from build123d import *

# Parameters (mm, degrees)
F1_DEPTH = 11
F2_DEPTH = 8
F3_DEPTH = 4.5


# Not quite as in the source:
# - ends of sketch curves that miss each other by under 0.0002 mm in the source are joined
# - a feature names something its author has since deleted; it is built from what else it names


with BuildPart() as f1:
    # F0 (on Top) → F1 (new body)
    with BuildSketch(Plane.XY):
        with BuildLine():
            ThreePointArc((-3.905e-06, -110), (9.5871245695, -109.5814174141), (19.1012892866, -108.3288546399))
            Line((19.1012892866, -108.3288546399), (18.1462248222, -102.9124119079))
            ThreePointArc((18.1462248222, -102.9124119079), (9.107768341, -104.1023465434), (-3.7098e-06, -104.5))
            Line((-3.7098e-06, -104.5), (-3.905e-06, -110))
        make_face()
        with BuildLine():
            Line((-18.1462345662, -102.9124101898), (-19.1012995434, -108.3288528313))
            ThreePointArc((-19.1012995434, -108.3288528313), (-9.5871336473, -109.5814166199), (-3.905e-06, -110))
            Line((-3.905e-06, -110), (-3.7098e-06, -104.5))
            ThreePointArc((-3.7098e-06, -104.5), (-9.107776965, -104.1023457889), (-18.1462345662, -102.9124101898))
        make_face()
    extrude(amount=F1_DEPTH)

    # F0 (on Top) → F2 (join)
    with BuildSketch(Plane.XY):
        with BuildLine():
            Line((-14.1061584567, -80), (-18.1462345662, -102.9124101898))
            ThreePointArc((-18.1462345662, -102.9124101898), (-9.107776965, -104.1023457889), (-3.7098e-06, -104.5))
            Line((-3.7098e-06, -104.5), (-3.673e-06, -103.4654280496))
            ThreePointArc((-3.673e-06, -103.4654280496), (-3.8705432222, -101.8678665034), (-5.4745569582, -97.999996388))
            Line((-5.4745569582, -97.999996388), (-5.4745569582, -85.9715496865))
            ThreePointArc((-5.4745569582, -85.9715496865), (-3.6975375335, -82.4283616447), (-2.8755e-06, -81))
            Line((-2.8755e-06, -81), (-2.84e-06, -80))
            Line((-2.84e-06, -80), (-14.1061584567, -80))
        make_face()
        with BuildLine():
            ThreePointArc((-3.7098e-06, -104.5), (9.107768341, -104.1023465434), (18.1462248222, -102.9124119079))
            Line((18.1462248222, -102.9124119079), (14.1061506466, -80))
            Line((14.1061506466, -80), (-2.84e-06, -80))
            Line((-2.84e-06, -80), (-2.8755e-06, -81))
            ThreePointArc((-2.8755e-06, -81), (3.6975315365, -82.4283617759), (5.4745508166, -85.9715496865))
            Line((5.4745508166, -85.9715496865), (5.4563215634, -97.999996388))
            ThreePointArc((5.4563215634, -97.999996388), (3.8587524181, -101.8614219128), (-3.673e-06, -103.4654280496))
            Line((-3.673e-06, -103.4654280496), (-3.7098e-06, -104.5))
        make_face()
    extrude(amount=F2_DEPTH)

    # F0 (on Top) → F3 (join)
    with BuildSketch(Plane.XY):
        with BuildLine():
            ThreePointArc((-5.4745569582, -97.999996388), (-3.8705432222, -101.8678665034), (-3.673e-06, -103.4654280496))
            Line((-3.673e-06, -103.4654280496), (-3.5722e-06, -100.6249805656))
            ThreePointArc((-3.5722e-06, -100.6249805656), (-1.862784569, -99.858636786), (-2.6341168729, -97.9979158754))
            Line((-2.6341168729, -97.9979158754), (-2.6250022463, -86.4979194874))
            ThreePointArc((-2.6250022463, -86.4979194874), (-1.8554226203, -84.6431092399), (-2.9776e-06, -83.875))
            Line((-2.9776e-06, -83.875), (-2.8755e-06, -81))
            ThreePointArc((-2.8755e-06, -81), (-3.6975375335, -82.4283616447), (-5.4745569582, -85.9715496865))
            Line((-5.4745569582, -85.9715496865), (-5.4745569582, -97.999996388))
        make_face()
        with BuildLine():
            Line((-3.5722e-06, -100.6249805656), (-3.673e-06, -103.4654280496))
            ThreePointArc((-3.673e-06, -103.4654280496), (3.8587524181, -101.8614219128), (5.4563215634, -97.999996388))
            Line((5.4563215634, -97.999996388), (5.4745508166, -85.9715496865))
            ThreePointArc((5.4745508166, -85.9715496865), (3.6975315365, -82.4283617759), (-2.8755e-06, -81))
            Line((-2.8755e-06, -81), (-2.9776e-06, -83.875))
            ThreePointArc((-2.9776e-06, -83.875), (1.8561522628, -84.6438447323), (2.6249969292, -86.5))
            ThreePointArc((2.6249969292, -86.5), (2.6249967231, -86.5010402564), (2.6249961047, -86.5020805126))
            Line((2.6249961047, -86.5020805126), (2.6158831271, -97.9999963886))
            ThreePointArc((2.6158831271, -97.9999963886), (2.6158820965, -98.0010366444), (2.6158814781, -98.0020769006))
            ThreePointArc((2.6158814781, -98.0020769006), (1.8495227006, -99.8536632596), (-3.5722e-06, -100.6249805656))
        make_face()
    extrude(amount=F3_DEPTH)


solid = f1.part
Geometry: final body of the model. Coordinates: model frame, mm. A direction names the side the tool comes from. Give positions to 0.01 mm unless a question says otherwise; leave off trailing zeros. Write each loop counter-clockwise with the first axis right and the second up, starting at its lowest first coordinate (ties: lowest second). Pieces come first, ordered by that corner, then holes. Notation, with made-up numbers: (28.25, -28.5) - (36.25, -28.5) arc R23 cw to (36.25, -15.5) - close; hole circle Ø5 at (47, -8). An arc over 180 degrees is marked (long way). Return JSON: item names as keys, results as strings. Group by question number.
1) Section A-A on y = -85.5. Return the cut outline in (x, z), plus the area to 3 significant figures.
2) Line query: line 1 (Z direction, x = 12, y = -103.5); line 2 (X direction, y = -100, z = 3.25); line 3 (Z direction, x = 3, y = -94). Output: solid intervals per line, ascending.
3) Set-up query: faces 1 (the flat face through (0, -80, 4)), 2 (the flat face through (8, -92, 8)), 3 (the flat face through (4, -92, 4.5)). Return all of +Z, -Z, +X, -X, +Y, -Y with unobstructed straight access to the full face (end or side cutting, diameter ignored); none if empty.
4) Section C-C on z = 8.5. Return the cut outline in (x, y), plus the area to 3 significant figures.
5) Section D-D on y = -104. Return the cut outline in (x, z), plus the area to 3 significant figures.
6) Section B-B on z = 6.25. Return the cut outline in (x, y), plus the area to 3 significant figures.
7) Mould query, pull axis X, two halves, no side actions, for faces 4 (the flat face through (0, -106, 11)), 5 (the flat face through (-5.475, -92, 6)). Classes: released by +X, released by -X, zero draft, split by the parting line, or undercut.
8) First-contact query: P1, Ø12, axis at x = 1.5, y = -89.5, coming from the +Z side; P2, Ø1, axis at y = -93, z = 8, coming from the +X side; P3, Ø4, axis at y = -92.5, z = 5.5, coming from the +X side; P4, Ø3, axis at y = -92.5, z = 10, coming from the +X side. Flat tips, straight axial feed; report the tip coordinate or a pass-through.
Filled in:
{
 "1": {"outline": "(-15.08, 0) - (-2.43, 0) - (-2.43, 4.5) - (-5.41, 4.5) - (-5.41, 8) - (-15.08, 8) - close; (2.43, 0) - (15.08, 0) - (15.08, 8) - (5.41, 8) - (5.41, 4.5) - (2.43, 4.5) - close", "area": "182 mm^2"},
 "2": {"line 1": "z = 0 to 8", "line 2": "x = -17.63 to -1.71, 1.69 to 17.63", "line 3": "z = 0 to 4.5"},
 "3": {"face 1": "+Z, -Z, +X, -X, +Y", "face 2": "+Z, +Y", "face 3": "+Z"},
 "4": {"outline": "(-19.1, -108.33) arc R110 ccw to (19.1, -108.33) - (18.15, -102.91) arc R104.5 cw to (-18.15, -102.91) - close", "area": "206 mm^2"},
 "5": {"outline": "(-18.34, 0) - (18.34, 0) - (18.34, 11) - (10.21, 11) - (10.21, 8) - (-10.21, 8) - (-10.21, 11) - (-18.34, 11) - close", "area": "342 mm^2"},
 "6": {"outline": "(-19.1, -108.33) arc R110 ccw to (19.1, -108.33) - (14.11, -80) - (-14.11, -80) - close; hole (-5.47, -98) arc R5.47 ccw to (5.46, -98) - (5.47, -85.97) arc R5.5 ccw to (-5.47, -85.97) - close", "area": "763 mm^2"},
 "7": {"face 4": "zero draft", "face 5": "undercut"},
 "8": {"P1": "stops at z = 8", "P2": "stops at x = 16.49", "P3": "stops at x = 16.66", "P4": "passes through"}
}
